Source: CAD feature listing. Evaluate the final solid. Frame: model axes, mm. Round coordinates to 2 decimals unless told otherwise and drop trailing zeros. Write each loop counter-clockwise with the first axis right and the second up, starting at its lowest first coordinate (ties: lowest second). Pieces come first, ordered by that corner, then holes. Notation, with made-up numbers: M 31.25,-17 L 36.25,-17 A7 cw 36.25,-4 Z; hole C 1,-1.5 d8. An arc over 180 degrees is marked long. Put each result on its own line as item: value. Start each with the question number.
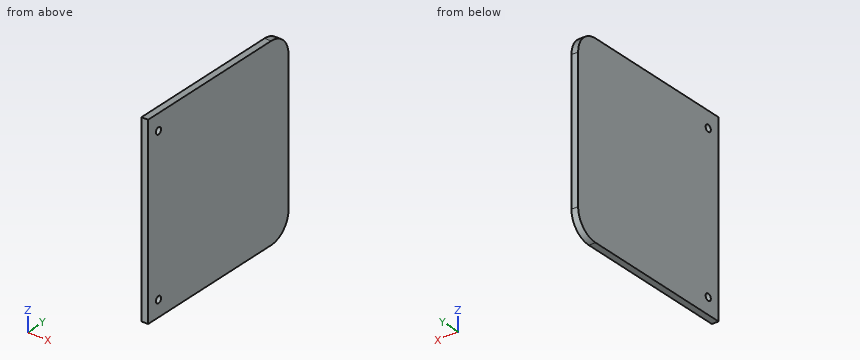
Autodesk Inventor part; units mm, degrees
ref_plane "Work Plane1" through (98.965, -88.9, 88.0899) normal (0, 0, -1) x (0, 1, 0)
ref_plane "Work Plane2" through (0, 0, 90.0899) normal (-1, 0, 0) x (0, 0, 1)
ref_plane "YZ Plane" through (0, 0, 0) normal (1, 0, 0) x (0, 1, 0)
sketch "Sketch1" plane through (0, 0, 0) normal (0, 0, 1) x (1, 0, 0)
  line L0 (104.68, -86.36) -> (104.68, -10.7)
  line L1 (101.505, -86.36) -> (104.68, -86.36)
  line L2 (148.8666, 2) -> (0, 2)
  line L3 (0, 0) -> (171.285, 0)
  line L4 (104.68, -86.36) -> (101.505, -86.36)
  line L5 (101.505, -86.36) -> (101.505, 16.1032)
  line L6 (101.505, 16.1032) -> (104.68, 16.1032)
  line L7 (104.68, 16.1032) -> (104.68, -86.36)
  dimension "d0" = 3.175
ref_plane "Work Plane1" through (98.965, -88.9, 88.0899) normal (0, 0, -1) x (0, 1, 0)
extrude "Extrusion1" add sketch "Sketch1" along normal up to surface (88.0899 mm away)
ref_plane "Work Plane2" through (0, 0, 90.0899) normal (-1, 0, 0) x (0, 0, 1)
sketch "Sketch2" plane through (0, 0, 90.0899) normal (-1, 0, 0) x (0, 0, 1)
  arc A0 (-79.3899, 2) -> (-92.0899, -10.7) centre (-79.3899, -10.7) ccw
  line L0 (-79.3899, 2) -> (-12.7, 2)
  arc A1 (0, -10.7) -> (-12.7, 2) centre (-12.7, -10.7) ccw
  line L1 (0, -10.7) -> (0, -82.9)
  arc A2 (0, -82.9) -> (2, -84.9) centre (2, -82.9) ccw
  line L2 (2, -84.9) -> (6.985, -84.9)
  line L3 (6.985, -84.9) -> (6.985, -88.9)
  line L4 (6.985, -88.9) -> (3.5017, -88.9)
  arc A3 (2.4019, -88.265) -> (3.5017, -88.9) centre (3.5017, -87.63) ccw
  arc A4 (2.4019, -88.265) -> (0.2021, -88.265) centre (1.302, -88.9) ccw
  arc A5 (-0.8977, -88.9) -> (0.2021, -88.265) centre (-0.8977, -87.63) ccw
  line L5 (-0.8977, -88.9) -> (-2, -88.9)
  line L6 (-2, -88.9) -> (-2, -10.7)
  arc A6 (-2, -10.7) -> (-12.7, 0) centre (-12.7, -10.7) ccw
  line L7 (-12.7, 0) -> (-79.3899, 0)
  arc A7 (-79.3899, 0) -> (-90.0899, -10.7) centre (-79.3899, -10.7) ccw
  line L8 (-90.0899, -10.7) -> (-90.0899, -88.9)
  line L9 (-90.0899, -88.9) -> (-91.1922, -88.9)
  arc A8 (-92.2921, -88.265) -> (-91.1922, -88.9) centre (-91.1922, -87.63) ccw
  arc A9 (-92.2921, -88.265) -> (-94.4918, -88.265) centre (-93.3919, -88.9) ccw
  arc A10 (-95.5916, -88.9) -> (-94.4918, -88.265) centre (-95.5916, -87.63) ccw
  line L10 (-95.5916, -88.9) -> (-99.0749, -88.9)
  line L11 (-99.0749, -88.9) -> (-99.0749, -84.9)
  line L12 (-99.0749, -84.9) -> (-94.0899, -84.9)
  arc A11 (-94.0899, -84.9) -> (-92.0899, -82.9) centre (-94.0899, -82.9) ccw
  line L13 (-92.0899, -82.9) -> (-92.0899, -10.7)
  line L14 (-2, -88.9) -> (-90.0899, -88.9)
  point P0 (-90.0899, 0)
extrude "Extrusion2" cut sketch "Sketch2" against normal through all contours L8 A7 L7 A6 L6 L14 keep common part
sketch "Sketch3" plane through (101.505, -86.36, 0) normal (-1, 0, 0) x (0, 0, 1)
  line L0 (0, 0) -> (0, 75.66)
  line L1 (0, 0) -> (88.0899, 0)
  line L2 (88.0899, 75.66) -> (88.0899, 0)
  circle A0 centre (7.62, 6.35) radius 1.5875
  circle A1 centre (80.4699, 6.35) radius 1.5875
  line L3 (7.62, 6.35) -> (67.6256, 6.35) construction
  point P0 (0, 86.36)
  dimension "d5" = 3.175
  dimension "d6" = 3.175
  dimension "d7" = 6.35
  dimension "d9" = 7.62
  dimension "d10" = 7.62
extrude "Extrusion3" cut sketch "Sketch3" against normal through all
equation "\"d10\" = d9"
properties part number "Divider"
(1) Ray query, line 1 along Z through (x, y) = (103.7, -80.01); line 2 along Z through (x, y) = (104.4, -81); line 3 along Y through (x, z) = (102.8, 7.62). Return the intervals inside material, ascending.
(2) Contact query for a flat-ended pin moving along its axis: P1, Ø1.9, axis at y = -80.01, z = 7.62, coming from the -X side. Output: stop coordinate, or through.
(3) Section query A-A (y = -80.01). Return loops of the section in (x, z) (1 decimal).
(4) Section query B-B (z = 7.62). Return loops of the section in (x, y) (1 decimal), and give its area (3 significant figures).
Entries:
1. line 1: 0 to 6.03, 9.21 to 78.88, 82.06 to 88.09
1. line 2: 0 to 6.38, 8.86 to 79.23, 81.71 to 88.09
1. line 3: -86.36 to -81.6, -78.42 to -0.45
2. P1: through
3. outline: M 101.5,0 L 104.7,0 L 104.7,6 L 101.5,6 Z; M 101.5,9.2 L 104.7,9.2 L 104.7,78.9 L 101.5,78.9 Z; M 101.5,82.1 L 104.7,82.1 L 104.7,88.1 L 101.5,88.1 Z
4. outline: M 101.5,-86.4 L 104.7,-86.4 L 104.7,-81.6 L 101.5,-81.6 Z; M 101.5,-78.4 L 104.7,-78.4 L 104.7,-0.5 L 101.5,-0.5 Z
4. area: 263 mm2
